Geometry check sheet. Reference: the model listing, model coordinates, mm. Give positions to 0.01 mm unless a question says otherwise; leave off trailing zeros. Order: outer loops, then holes, each group sorted by start corner. A loop starts at its lowest first (then second) coordinate and runs counter-clockwise, first axis right, second up. Notation, with made-up numbers: M 55,-22 L 98,-22 A16 ccw 98,5 Z; hole C 61.5,16.5 d4. An arc over 180 degrees is marked long. Answer as CSV lines item,"result".
from build123d import *

# Parameters (mm, degrees)
SKETCH1_W           = 384.714130078
SKETCH1_H           = 50.8
SKETCH1_R           = 14.3002
SKETCH1_R_2         = 2.0193
SKETCH1_R_3         = 2.54
BOSS_EXTRUDE1_DEPTH = 3.175
FILLET1_R           = 7.62


with BuildPart() as part:
    # Sketch1 → Boss-Extrude1 (new body)
    with BuildSketch(Plane.XY):
        with Locations((91.437616825, 0.672961839)):
            Rectangle(SKETCH1_W, SKETCH1_H)
        with Locations((-74.109858368, 0.672961839)):
            Circle(SKETCH1_R, mode=Mode.SUBTRACT)
        with Locations((14.028141632, 0.672961839)):
            Circle(SKETCH1_R, mode=Mode.SUBTRACT)
        with Locations((259.138141632, 0.672961839)):
            Circle(SKETCH1_R, mode=Mode.SUBTRACT)
        with Locations((39.592109109, 0.662961839)):
            Circle(SKETCH1_R_2, mode=Mode.SUBTRACT)
        with Locations((32.152621351, -17.297550403)):
            Circle(SKETCH1_R_2, mode=Mode.SUBTRACT)
        with Locations((-3.768403133, -17.297550403)):
            Circle(SKETCH1_R_2, mode=Mode.SUBTRACT)
        with Locations((32.152621351, 18.623474081)):
            Circle(SKETCH1_R_2, mode=Mode.SUBTRACT)
        with Locations((-11.207890891, 0.662961839)):
            Circle(SKETCH1_R_2, mode=Mode.SUBTRACT)
        with Locations((-29.885519869, 7.289574438)):
            Circle(SKETCH1_R_3, mode=Mode.SUBTRACT)
        with Locations((-29.885519869, -5.410425562)):
            Circle(SKETCH1_R_3, mode=Mode.SUBTRACT)
        with Locations((-17.185519869, 7.289574438)):
            Circle(SKETCH1_R_3, mode=Mode.SUBTRACT)
        with Locations((-17.185519869, -5.410425562)):
            Circle(SKETCH1_R_3, mode=Mode.SUBTRACT)
        with Locations((-17.185519869, -18.110425562)):
            Circle(SKETCH1_R_3, mode=Mode.SUBTRACT)
        with Locations((-17.185519869, 19.989574438)):
            Circle(SKETCH1_R_3, mode=Mode.SUBTRACT)
        with Locations((-30.066807854, 19.989574438)):
            Circle(SKETCH1_R_3, mode=Mode.SUBTRACT)
        with Locations((33.614480131, -5.410425562)):
            Circle(SKETCH1_R_3, mode=Mode.SUBTRACT)
        with Locations((33.614480131, 7.289574438)):
            Circle(SKETCH1_R_3, mode=Mode.SUBTRACT)
        with Locations((59.014480131, -5.410425562)):
            Circle(SKETCH1_R_3, mode=Mode.SUBTRACT)
        with Locations((59.014480131, 7.289574438)):
            Circle(SKETCH1_R_3, mode=Mode.SUBTRACT)
        with Locations((46.314480131, 7.289574438)):
            Circle(SKETCH1_R_3, mode=Mode.SUBTRACT)
        with Locations((46.314480131, -5.410425562)):
            Circle(SKETCH1_R_3, mode=Mode.SUBTRACT)
        with Locations((46.314480131, -18.110425562)):
            Circle(SKETCH1_R_3, mode=Mode.SUBTRACT)
        with Locations((58.833192146, -18.110425562)):
            Circle(SKETCH1_R_3, mode=Mode.SUBTRACT)
        with Locations((71.533192146, -18.110425562)):
            Circle(SKETCH1_R_3, mode=Mode.SUBTRACT)
        with Locations((71.533192146, -5.410425562)):
            Circle(SKETCH1_R_3, mode=Mode.SUBTRACT)
        with Locations((71.533192146, 7.289574438)):
            Circle(SKETCH1_R_3, mode=Mode.SUBTRACT)
        with Locations((71.533192146, 19.989574438)):
            Circle(SKETCH1_R_3, mode=Mode.SUBTRACT)
        with Locations((58.833192146, 19.989574438)):
            Circle(SKETCH1_R_3, mode=Mode.SUBTRACT)
        with Locations((46.314480131, 19.989574438)):
            Circle(SKETCH1_R_3, mode=Mode.SUBTRACT)
        with Locations((20.733192146, 19.989574438)):
            Circle(SKETCH1_R_3, mode=Mode.SUBTRACT)
        with Locations((8.033192146, 19.989574438)):
            Circle(SKETCH1_R_3, mode=Mode.SUBTRACT)
        with Locations((-4.666807854, 19.989574438)):
            Circle(SKETCH1_R_3, mode=Mode.SUBTRACT)
        with Locations((20.733192146, -18.110425562)):
            Circle(SKETCH1_R_3, mode=Mode.SUBTRACT)
        with Locations((8.033192146, -18.110425562)):
            Circle(SKETCH1_R_3, mode=Mode.SUBTRACT)
        with Locations((-30.066807854, -18.110425562)):
            Circle(SKETCH1_R_3, mode=Mode.SUBTRACT)
        with Locations((-42.766807854, -18.110425562)):
            Circle(SKETCH1_R_3, mode=Mode.SUBTRACT)
        with Locations((-42.766807854, 19.989574438)):
            Circle(SKETCH1_R_3, mode=Mode.SUBTRACT)
        with Locations((-42.766807854, 7.289574438)):
            Circle(SKETCH1_R_3, mode=Mode.SUBTRACT)
        with Locations((-42.766807854, -5.410425562)):
            Circle(SKETCH1_R_3, mode=Mode.SUBTRACT)
    extrude(amount=BOSS_EXTRUDE1_DEPTH)

    # Fillet1
    fillet1_edges = [part.edges().sort_by_distance(p)[0] for p in [
        (-100.919448214, 26.072961839, 1.5875),
        (283.794681864, 26.072961839, 1.5875),
        (283.794681864, -24.727038161, 1.5875),
        (-100.919448214, -24.727038161, 1.5875),
    ]]
    fillet(fillet1_edges, radius=FILLET1_R)


solid = part.part
(1) Gauge pin test, flat end, axial feed: P1, Ø3, axis at x = -17.19, y = -5.41, coming from the -Z side. Record the tip position at first contact, or that the pin passes through.
The answers:
P1,"passes through"
(2) Material ranges on line 1 (X direction, y = 3, z = 0.3); line 2 (X direction, y = -10, z = 1.85); line 3 (X direction, y = 2.5, z = 0.65), recorded low to high.
The answers:
line 1,"x = -100.92 to -88.22, -60 to -0.08, 28.14 to 245.03, 273.25 to 283.79"
line 2,"x = -100.92 to -83.63, -64.59 to 4.51, 23.55 to 249.62, 268.66 to 283.79"
line 3,"x = -100.92 to -88.29, -59.93 to -12.05, -10.37 to -0.15, 28.21 to 38.75, 40.43 to 244.96, 273.32 to 283.79"
(3) Section check A-A on x = -75. Enter the section's corners in (y, z) (1 decimal).
The answers:
outline,"M -24.7,0 L -13.6,0 L -13.6,3.2 L -24.7,3.2 Z; M 14.9,0 L 26.1,0 L 26.1,3.2 L 14.9,3.2 Z"
(4) Draft check along Y on faces 1 (the face through (-98.747, -22.436, 1.61)), 2 (the face through (-98.75, 23.78, 1.61)), 3 (the face through (27.668, 4.968, 1.565)), 4 (the face through (89, 1, 3.175)). Enter one of: +Y half, -Y half, draft (parallel to the pull), parting line (faces both ways), or undercut.
The answers:
face 1,"-Y half"
face 2,"+Y half"
face 3,"undercut"
face 4,"draft"
(5) Section check B-B on z = 1.4. State how many separate pieces and enclosed holes the cut face has, then the cut area to 3 significant figures.
The answers:
separate pieces,"1"
enclosed holes,"39"
area,"16,900 mm2"
